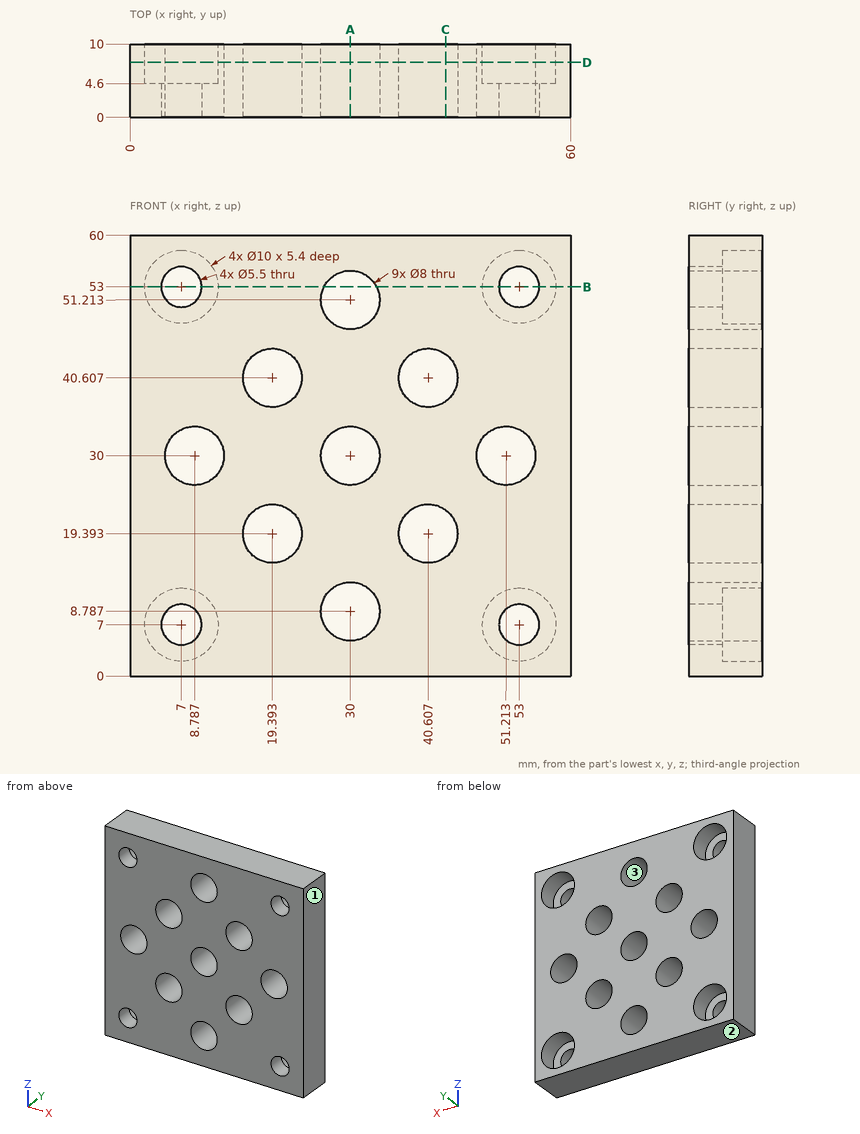
Job drawing, mm, ordinate dimensions from the low corner. One solid piece. Give positions to 0.01 mm unless a question says otherwise; leave off trailing zeros. Write each loop counter-clockwise with the first axis right and the second up, starting at its lowest first coordinate (ties: lowest second). Pieces come first, ordered by that corner, then holes. Notation, with made-up numbers: M 83,88 L 141,88 A28 ccw 141,117 Z; hole C 23.5,74 d11. An arc over 180 degrees is marked long. Put each result on its own line as item: value. Start each with the question number.
(1) Band-saw the part on B-B, the plane z = 53. Write the cut outline in (x, y).
(2) Band-saw the part on C-C, the plane x = 43. Write the cut outline in (y, z), and give its area (3 significant figures).
(3) Flat gauge pins, fed straight in: pin 1 Ø6.5 at (x, z) = (19.39, 19.39) entering from -Y; pin 2 Ø5 at (x, z) = (52.5, 5.5) entering from +Y. Where does each tip first touch, or does it go through?
(4) Band-saw the part on A-A, the plane x = 30. Write the cut outline in (y, z), and give its area (3 significant figures).
(5) Mould opens along X. For the marked faces 1, 2 and 3 say: +X half, -X half, draft (parallel to the pull), parting line (faces both ways), or undercut.
(6) Band-saw the part on D-D, the plane y = 7.5. Give the number of separate pieces and of enclosed holes in the cut face, and give its area (3 significant figures).
(7) Probe L1, parallel to X at y = 5, z = 23 (1 decimal); L2, parallel to Z at x = 3, y = 8.5; L3, parallel to Z at x = 30, y = 4. List the from-to ranges inside material, lowest first.
Response values:
1. outline: M 0,0 L 4.25,0 L 4.25,4.6 L 2,4.6 L 2,10 L 0,10 Z; M 9.75,0 L 26.42,0 L 26.42,10 L 12,10 L 12,4.6 L 9.75,4.6 Z; M 33.58,0 L 50.25,0 L 50.25,4.6 L 48,4.6 L 48,10 L 33.58,10 Z; M 55.75,0 L 60,0 L 60,10 L 58,10 L 58,4.6 L 55.75,4.6 Z
2. outline: M 0,0 L 10,0 L 10,16.19 L 0,16.19 Z; M 0,22.6 L 10,22.6 L 10,37.4 L 0,37.4 Z; M 0,43.81 L 10,43.81 L 10,60 L 0,60 Z
2. area: 472 mm2
3. pin 1: passes through
3. pin 2: stops at y = 4.6
4. outline: M 0,0 L 10,0 L 10,4.79 L 0,4.79 Z; M 0,12.79 L 10,12.79 L 10,26 L 0,26 Z; M 0,34 L 10,34 L 10,47.21 L 0,47.21 Z; M 0,55.21 L 10,55.21 L 10,60 L 0,60 Z
4. area: 360 mm2
5. face 1: +X half
5. face 2: draft
5. face 3: undercut
6. separate pieces: 1
6. enclosed holes: 13
6. area: 2,830 mm2
7. L1: x = 0 to 17.7, 21.1 to 38.9, 42.3 to 60
7. L2: z = 0 to 4, 10 to 50, 56 to 60
7. L3: z = 0 to 4.79, 12.79 to 26, 34 to 47.21, 55.21 to 60
